from build123d import *

# Parameters (mm, degrees)
BOSS_EXTRUDE1_DEPTH      = 2
BOSS_EXTRUDE1_DEPTH_BACK = 2
SKETCH1_R                = 5
SKETCH1_R_2              = 2
SKETCH2_R                = 4
SKETCH2_R_2              = 3
CUT_EXTRUDE1_DEPTH       = 0.6
CHAMFER1_SIZE            = 0.1


with BuildPart() as part:
    # Sketch1 → Boss-Extrude1 (new, two sides: drawn at the far end of the back side and taken through both)
    with BuildSketch(Plane(origin=(0, 0, 0), x_dir=(1, 0, 0), z_dir=(0, 1, 0)).offset(-BOSS_EXTRUDE1_DEPTH_BACK)):
        with Locations(Location((0, 0, 0), (0, 0, 270))):
            Circle(SKETCH1_R)
        with Locations(Location((0, 0, 0), (0, 0, 270))):
            Circle(SKETCH1_R_2, mode=Mode.SUBTRACT)
    extrude(amount=BOSS_EXTRUDE1_DEPTH + BOSS_EXTRUDE1_DEPTH_BACK)

    # Sketch2 → Cut-Extrude1 (cut)
    with BuildSketch(Plane(origin=(0, 2, 0), x_dir=(1, 0, 0), z_dir=(0, 1, 0))):
        with Locations(Location((0, 0, 0), (0, 0, 270))):
            Circle(SKETCH2_R)
        with Locations(Location((0, 0, 0), (0, 0, 270))):
            Circle(SKETCH2_R_2, mode=Mode.SUBTRACT)
    cut_extrude1 = extrude(amount=-CUT_EXTRUDE1_DEPTH, mode=Mode.SUBTRACT)

    # Mirror2: Cut-Extrude1 across plane
    add(cut_extrude1.mirror(Plane.ZX), mode=Mode.SUBTRACT)

    # Chamfer1
    chamfer1_edges = [part.edges().sort_by_distance(p)[0] for p in [
        (0, -2, -5),
        (0, 2, -5),
    ]]
    chamfer(chamfer1_edges, length=CHAMFER1_SIZE)


solid = part.part
Check sheet for the modelled part. Datum: model origin and axes. Units: mm. A direction names the side the tool comes from. Round coordinates to 2 decimals unless told otherwise and drop trailing zeros. Write each loop counter-clockwise with the first axis right and the second up, starting at its lowest first coordinate (ties: lowest second). Pieces come first, ordered by that corner, then holes. Notation, with made-up numbers: (51, 81) - (98, 81) arc R24 ccw to (98, 98) - close; hole circle Ø3 at (-10, -31.75). An arc over 180 degrees is marked (long way). Return JSON: item names as keys, results as strings.
Q1. Cross-section at C-C (y = -1.7). Record the boundary of the cut face in (x, z).
Returned:
{"outline": "circle Ø10 at (0, 0); circle Ø6 at (0, 0); hole circle Ø8 at (0, 0); hole circle Ø4 at (0, 0)"}
Q2. Draft check along X on faces 4 (the cylindrical face through (-3.905, 1.704, -0.867)), 5 (the flat face through (-4, -2, -2)), 6 (the cylindrical face through (-4.88, -0.03, -1.08)). Enter one of: released by +X, released by -X, zero draft, split by the parting line, or undercut.
Returned:
{"face 4": "undercut", "face 5": "zero draft", "face 6": "split by the parting line"}
Q3. Scan lines: L1, parallel to X at y = -1.7, z = 0; L2, parallel to Z at x = -1.5, y = -1.5; L3, parallel to Z at x = 1, y = -1.6. Record each from-to range of solid material in increasing order. Write a range as from..to.
Returned:
{"L1": "x = -5..-4, -3..-2, 2..3, 4..5", "L2": "z = -4.77..-3.71, -2.6..-1.32, 1.32..2.6, 3.71..4.77", "L3": "z = -4.9..-3.87, -2.83..-1.73, 1.73..2.83, 3.87..4.9"}
Q4. Access from +Z, -Z, +X, -X, +Y, -Y to the whole of each face (thin tool, end or side, straight path). Record for faces 1 (the cylindrical face through (0.9, -1.7, 2.86)), 2 (the flat face through (3, 1.4, 1)), 3 (the flat face through (-1, 2, 2)).
Returned:
{"face 1": "-Y", "face 2": "+Y", "face 3": "+Z, -Z, +X, -X, +Y"}
Q5. Cross-section at B-B (z = 0). Record the boundary of the cut face in (x, y), then the cut area to 3 significant figures.
Returned:
{"outline": "(-5, -1.9) - (-4.9, -2) - (-4, -2) - (-4, -1.4) - (-3, -1.4) - (-3, -2) - (-2, -2) - (-2, 2) - (-3, 2) - (-3, 1.4) - (-4, 1.4) - (-4, 2) - (-4.9, 2) - (-5, 1.9) - close; (2, -2) - (3, -2) - (3, -1.4) - (4, -1.4) - (4, -2) - (4.9, -2) - (5, -1.9) - (5, 1.9) - (4.9, 2) - (4, 2) - (4, 1.4) - (3, 1.4) - (3, 2) - (2, 2) - close", "area": "21.6 mm²"}
Q6. Cross-section at A-A (x = 0). Record the boundary of the cut face in (y, z).
Returned:
{"outline": "(-2, -4.9) - (-1.9, -5) - (1.9, -5) - (2, -4.9) - (2, -4) - (1.4, -4) - (1.4, -3) - (2, -3) - (2, -2) - (-2, -2) - (-2, -3) - (-1.4, -3) - (-1.4, -4) - (-2, -4) - close; (-2, 2) - (2, 2) - (2, 3) - (1.4, 3) - (1.4, 4) - (2, 4) - (2, 4.9) - (1.9, 5) - (-1.9, 5) - (-2, 4.9) - (-2, 4) - (-1.4, 4) - (-1.4, 3) - (-2, 3) - close"}
Q7. Cross-section at D-D (y = -0.2). Record the boundary of the cut face in (x, z).
Returned:
{"outline": "circle Ø10 at (0, 0); hole circle Ø4 at (0, 0)"}
Q8. Depth check by flat-ended pin: P1, Ø1, axis at x = 2.5, y = 1.5, coming from the -Z side; P2, Ø1, axis at y = -1.5, z = -3.5, coming from the -X side; P3, Ø2, axis at y = 0, z = 2, coming from the +X side. Enter the tip coordinate at first touch or a pass-through.
Returned:
{"P1": "stops at z = -4.58", "P2": "stops at x = -4", "P3": "stops at x = 4.9"}
